The model under review builds one solid part; all positions refer to its coordinate system, in mm. Face numbers are marked on the shaded views. A direction names the side the tool comes from. Give positions to 0.01 mm unless a question says otherwise; leave off trailing zeros. Order: outer loops, then holes, each group sorted by start corner. A loop starts at its lowest first (then second) coordinate and runs counter-clockwise, first axis right, second up. Notation, with made-up numbers: (39, -21) -> (54, -21) arc R22 ccw to (54, -7) -> close; hole circle Ø7 at (9, 38.5). An arc over 180 degrees is marked (long way). Use one line per item in the form item = value.
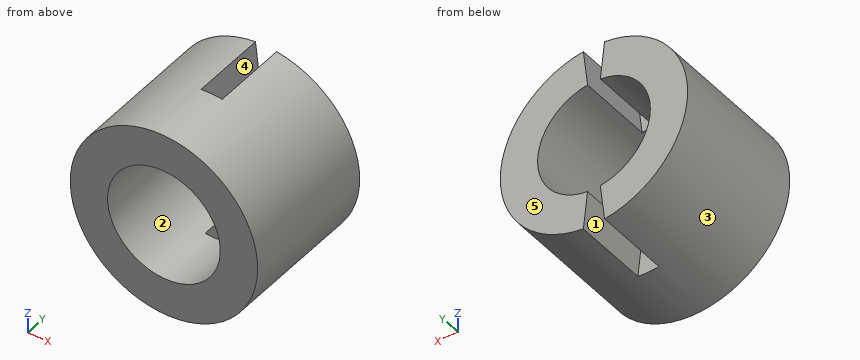
```python
from build123d import *

# Parameters (mm, degrees)
SKETCH1_R           = 10.05
SKETCH1_R_2         = 6.05
BOSS_EXTRUDE1_DEPTH = 15
CUT_EXTRUDE2_DEPTH  = 8


with BuildPart() as part:
    # Sketch1 → Boss-Extrude1 (new body)
    with BuildSketch(Plane(origin=(0, 0, 0), x_dir=(1, 0, 0), z_dir=(0, 1, 0))):
        with Locations(Location((0, 0, 0), (0, 0, 270))):
            Circle(SKETCH1_R)
        with Locations(Location((0, 0, 0), (0, 0, 270))):
            Circle(SKETCH1_R_2, mode=Mode.SUBTRACT)
    extrude(amount=BOSS_EXTRUDE1_DEPTH)

    # Sketch6 → Cut-Extrude2 (cut)
    with BuildSketch(Plane(origin=(0, 15, 0), x_dir=(1, 0, 0), z_dir=(0, 1, 0))):
        Polygon((-0.637272671, 5.61077026), (0.637272671, 5.61077026), (1.215708589, 10.703521268), (-1.215708589, 10.703521268), align=None)
        Polygon((-0.637272671, -5.61077026), (-1.215708589, -10.703521268), (1.215708589, -10.703521268), (0.637272671, -5.61077026), align=None)
    extrude(amount=-CUT_EXTRUDE2_DEPTH, mode=Mode.SUBTRACT)


solid = part.part
```
1. Add section B-B on x = 0. Give the boundary of the cut face in (y, z), then the cut area to 3 significant figures.
Values:
outline = (0, -10.05) -> (7, -10.05) -> (7, -6.05) -> (0, -6.05) -> close; (0, 6.05) -> (7, 6.05) -> (7, 10.05) -> (0, 10.05) -> close
area = 56.0 mm^2
2. Add section D-D on y = 4.75. Give the boundary of the cut face in (x, z).
Values:
outline = circle Ø20.1 at (0, 0); hole circle Ø12.1 at (0, 0)
3. For L1, parallel to X at y = 4.75, z = 0; L2, parallel to Z at x = 0.25, y = 4; L3, parallel to X at y = 9.5, z = 3, list the stretches that pass through material, from the lowest coordinate up.
Values:
L1 = -10.05 to -6.05, 6.05 to 10.05
L2 = -10.05 to -6.04, 6.04 to 10.05
L3 = -9.59 to -5.25, 5.25 to 9.59
4. For pin 1 Ø1.5 at (y, z) = (6, 3.5) entering from -X; pin 2 Ø0.7 at (x, z) = (0.5, 9) entering from +Y; pin 3 Ø1 at (x, y) = (-3, 2) entering from -Z, all flat-tipped, find the tip position at first contact; note any pin that passes through.
Values:
pin_1 = -9.67
pin_2 = 7
pin_3 = -9.73
5. Add section C-C on z = 8.75. Give the boundary of the cut face in (x, y).
Values:
outline = (-4.94, 0) -> (4.94, 0) -> (4.94, 15) -> (0.99, 15) -> (0.99, 7) -> (-0.99, 7) -> (-0.99, 15) -> (-4.94, 15) -> close
6. The part is to be moulded in two halves that separate along X. For the marked faces 3, 4 and 5, say which applies: +X half, -X half, draft (parallel to the pull), parting line (faces both ways), or undercut.
Values:
face_3 = parting line
face_4 = undercut
face_5 = draft
7. Tool access review of the marked faces 1 and 2: name each direction out of +Z, -Z, +X, -X, +Y, -Y from which nothing blocks a thin tool from reaching the whole face with its end or side.
Values:
face_1 = -Z, +Y
face_2 = +Y, -Y
